Verification items for the finished model (mm, model axes). A direction names the side the tool comes from. Coordinates: 2 decimals unless noted, no trailing zeros. Order: outer loops, then holes, each group sorted by start corner. A loop starts at its lowest first (then second) coordinate and runs counter-clockwise, first axis right, second up. Notation, with made-up numbers: (29, 8.25) -> (56, 8.25) arc R17 ccw to (56, 41.25) -> close; hole circle Ø9 at (10, 5.25). An arc over 180 degrees is marked (long way). Answer as CSV lines item,"result".
```python
from build123d import *

# Parameters (mm, degrees)
F1_DEPTH = 40
F3_DEPTH = 40
F5_DEPTH = 20
F6_R     = 2


with BuildPart() as f1:
    # F0 (on Front) → F1 (new body)
    with BuildSketch(Plane.XZ):
        with BuildLine():
            Line((-21, -10.8208951545), (0, -10.8208951545))
            Line((0, -10.8208951545), (21, -10.8208951545))
            ThreePointArc((21, -10.8208951545), (25.8896090165, -9.8248824487), (30, -6.9955709409))
            ThreePointArc((30, -6.9955709409), (32.2508823643, -3.7676966034), (33.3867108999, 0))
            ThreePointArc((33.3867108999, 0), (30.4137880412, 9.9028871089), (21, 14.1791048455))
            Line((21, 14.1791048455), (0, 14.1791048455))
            Line((0, 14.1791048455), (-21, 14.1791048455))
            ThreePointArc((-21, 14.1791048455), (-30.4137880412, 9.9028871089), (-33.3867108999, 0))
            ThreePointArc((-33.3867108999, 0), (-32.2508823643, -3.7676966034), (-30, -6.9955709409))
            ThreePointArc((-30, -6.9955709409), (-25.8896090165, -9.8248824487), (-21, -10.8208951545))
        make_face()
        with BuildLine():
            ThreePointArc((33.3867108999, 0), (32.2508823643, -3.7676966034), (30, -6.9955709409))
            Line((30, -6.9955709409), (35, -17.6733862609))
            Line((35, -17.6733862609), (35, -22.8208951545))
            Line((35, -22.8208951545), (50, -22.8208951545))
            Line((50, -22.8208951545), (50, -18.8208951545))
            Line((50, -18.8208951545), (42.8475700319, -18.8208951545))
            Line((42.8475700319, -18.8208951545), (33.3867108999, 0))
        make_face()
        with BuildLine():
            Line((-35, -17.6733862609), (-30, -6.9955709409))
            ThreePointArc((-30, -6.9955709409), (-32.2508823643, -3.7676966034), (-33.3867108999, 0))
            Line((-33.3867108999, 0), (-42.8475700319, -18.8208951545))
            Line((-42.8475700319, -18.8208951545), (-50, -18.8208951545))
            Line((-50, -18.8208951545), (-50, -22.8208951545))
            Line((-50, -22.8208951545), (-35, -22.8208951545))
            Line((-35, -22.8208951545), (-35, -17.6733862609))
        make_face()
    extrude(amount=F1_DEPTH)

    # F2 (on face) → F3 (join)
    with BuildSketch(Plane.XZ.offset(40)):
        with BuildLine():
            Line((21, 14.1791048455), (-21, 14.1791048455))
            ThreePointArc((-21, 14.1791048455), (-33.5, 1.6791048455), (-21, -10.8208951545))
            Line((-21, -10.8208951545), (21, -10.8208951545))
            ThreePointArc((21, -10.8208951545), (33.5, 1.6791048455), (21, 14.1791048455))
        make_face()
    extrude(amount=F3_DEPTH)

    # F4 (on face) + F2 (on face) → F5 (join)
    with BuildSketch(Plane(origin=(0, 0, 0), x_dir=(-1, 0, 0), z_dir=(0, 1, 0))):
        with BuildLine():
            Line((-21, -10.8208951545), (21, -10.8208951545))
            ThreePointArc((21, -10.8208951545), (33.5, 1.6791048455), (21, 14.1791048455))
            Line((21, 14.1791048455), (-21, 14.1791048455))
            ThreePointArc((-21, 14.1791048455), (-33.5, 1.6791048455), (-21, -10.8208951545))
        make_face()
    with BuildSketch(Plane.XZ.offset(40)):
        with BuildLine():
            Line((21, 14.1791048455), (-21, 14.1791048455))
            ThreePointArc((-21, 14.1791048455), (-33.5, 1.6791048455), (-21, -10.8208951545))
            Line((-21, -10.8208951545), (21, -10.8208951545))
            ThreePointArc((21, -10.8208951545), (33.5, 1.6791048455), (21, 14.1791048455))
        make_face()
    extrude(amount=F5_DEPTH, dir=(0, 1, 0))

    # F6
    f6_edges = [f1.edges().sort_by_distance(p)[0] for p in [
        (0, -80, 14.179105),
        (33.5, -80, 1.679105),
        (0, -80, -10.820895),
        (-33.5, -80, 1.679105),
    ]]
    fillet(f6_edges, radius=F6_R)


solid = f1.part
```
Item 1: Section check B-B, the plane x = 8. Record the boundary of the cut face in (y, z), plus the area to 3 significant figures.
Answer list:
outline,"(-80, -8.82) arc R2 ccw to (-78, -10.82) -> (20, -10.82) -> (20, 14.18) -> (-78, 14.18) arc R2 ccw to (-80, 12.18) -> close"
area,"2,500 mm2"
Item 2: Release check for a two-part mould opening along X. For faces 4 (the flat face through (38.183, -19.72, -9.542)), 5 (the flat face through (42, -20, -22.821)), 6 (the flat face through (-38.05, -19.72, -9.28)), 7 (the flat face through (0, -30, -10.821)) record: +X half, -X half, draft (parallel to the pull), parting line (faces both ways), or undercut.
Answer list:
face 4,"+X half"
face 5,"draft"
face 6,"-X half"
face 7,"undercut"
Item 3: Section check C-C, the plane y = -65.5. Record the boundary of the cut face in (x, z), plus the area to 3 significant figures.
Answer list:
outline,"(-21, -10.82) -> (21, -10.82) arc R12.5 ccw to (21, 14.18) -> (-21, 14.18) arc R12.5 ccw to start"
area,"1,540 mm2"
Item 4: Tool access check on faces 1 (the flat face through (46, -20, -18.821)), 2 (the flat face through (-32.535, -19.72, -12.409)), 3 (the flat face through (-38, -40, -14)). Record the directions out of +Z, -Z, +X, -X, +Y, -Y that give a thin tool (end or side, any length) a straight path to the whole face; none if there is none.
Answer list:
face 1,"+Z, +X, +Y, -Y"
face 2,"-Z, +Y, -Y"
face 3,"-Z, -X, -Y"
Item 5: Section check A-A, the plane y = -26. Record the boundary of the cut face in (x, z), plus the area to 3 significant figures.
Answer list:
outline,"(-50, -22.82) -> (-35, -22.82) -> (-35, -17.67) -> (-30, -7) arc R12.5 ccw to (-21, -10.82) -> (21, -10.82) arc R12.5 ccw to (30, -7) -> (35, -17.67) -> (35, -22.82) -> (50, -22.82) -> (50, -18.82) -> (42.85, -18.82) -> (33.39, 0) arc R12.5 ccw to (21, 14.18) -> (-21, 14.18) arc R12.5 ccw to (-33.39, 0) -> (-42.85, -18.82) -> (-50, -18.82) -> close"
area,"1,870 mm2"
Item 6: Depth check by flat-ended pin: pin 1 Ø2 at (x, y) = (-47.5, -19) entering from +Z; pin 2 Ø6 at (x, z) = (-37.5, -6) entering from -Y; pin 3 Ø8 at (y, z) = (-21.5, 7.5) entering from -X. Enter the tip coordinate at first touch or a pass-through.
Answer list:
pin 1,"z = -18.82"
pin 2,"y = -40"
pin 3,"x = -33.37"
Item 7: Thickness scan on line 1 (X direction, y = -0.5, z = -8); line 2 (Z direction, x = 16.5, y = -10); line 3 (Y direction, x = -37, z = -19.5). Record the ranges inside material, lowest first.
Answer list:
line 1,"-37.41 to -30.47, -28.91 to 28.91, 30.47 to 37.41"
line 2,"-10.82 to 14.18"
line 3,"-40 to 0"
